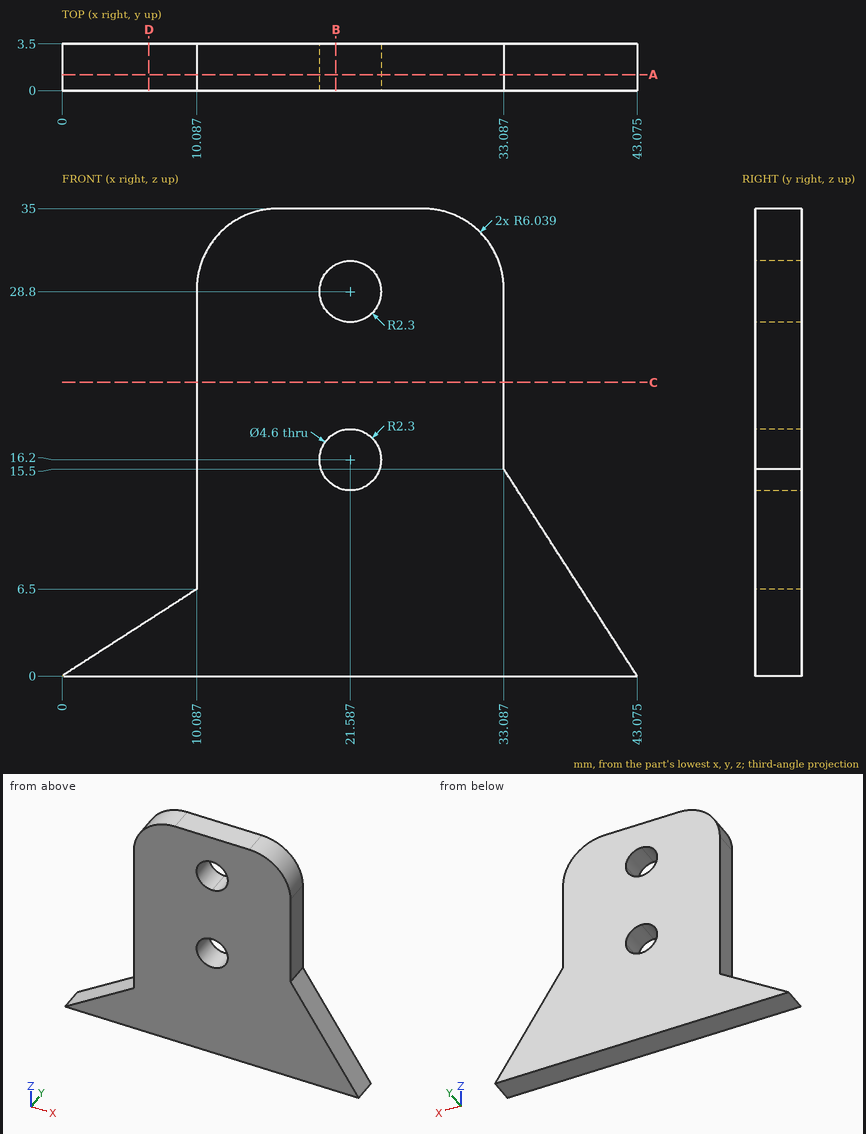
Answer from the drawing. Dimensions are ordinates in mm from the lowest x, y and z of the part. Give positions to 0.01 mm unless a question says otherwise; leave off trailing zeros. Loops run counter-clockwise (first coordinate to the right, second up) from the corner with the lowest first, then second, coordinate; pieces in that order, holes last. Notation, with made-up numbers: (52.5, 81) - (83.5, 81) arc R15 cw to (83.5, 100) - close; hole circle Ø9 at (-32.5, 16.25). An arc over 180 degrees is marked (long way). Answer as a JSON object with one key per item and string values.
1. A cutting plane is placed at D-D (x = 6.5). Write down the section's boundary in (y, z).
Determined:
{"outline": "(0, 0) - (3.5, 0) - (3.5, 4.19) - (0, 4.19) - close"}
2. A cutting plane is placed at C-C (z = 22). Write down the section's boundary in (x, y).
Determined:
{"outline": "(10.09, 0) - (33.09, 0) - (33.09, 3.5) - (10.09, 3.5) - close"}
3. A cutting plane is placed at B-B (x = 20.5). Write down the section's boundary in (y, z).
Determined:
{"outline": "(0, 0) - (3.5, 0) - (3.5, 14.17) - (0, 14.17) - close; (0, 18.23) - (3.5, 18.23) - (3.5, 26.77) - (0, 26.77) - close; (0, 30.83) - (3.5, 30.83) - (3.5, 35) - (0, 35) - close"}
4. Find the intervals of material crossed by L1, parallel to X at y = 2.6, z = 16.2; L2, parallel to X at y = 2.8, z = 14.5 (1 decimal); L3, parallel to Z at x = 20, y = 0.2 (1 decimal), in increasing order. Write a range as [from, to].
Determined:
{"L1": "[10.09, 19.29], [23.89, 33.09]", "L2": "[10.1, 20], [23.1, 33.7]", "L3": "[0, 14.5], [17.9, 27.1], [30.5, 35]"}
5. A cutting plane is placed at A-A (y = 1.2). Write down the section's boundary in (x, z) (1 decimal), then the cut area to 3 significant figures.
Determined:
{"outline": "(0, 0) - (43.1, 0) - (33.1, 15.5) - (33.1, 29) arc R6 ccw to (27, 35) - (16.1, 35) arc R6 ccw to (10.1, 29) - (10.1, 6.5) - close; hole (21.6, 18.5) arc R2.3 ccw (long way) to (23.9, 16.2) arc R2.3 ccw to start; hole (21.6, 26.5) arc R2.3 ccw to (23.9, 28.8) arc R2.3 ccw to (21.6, 31.1) arc R2.3 ccw to start", "area": "866 mm²"}
6. Flat-ended cylindrical pins translate along their axes: pin 1 Ø2 at (y, z) = (1.5, 28) entering from +X; pin 2 Ø1 at (y, z) = (1, 19) entering from -X. Find the tip coordinate at first contact, or state that the pin passes through.
Determined:
{"pin 1": "x = 33.09", "pin 2": "x = 10.09"}
